Can you work these out from the drawing? Everything is in mm from the part's minimum corner. Coordinates: 2 decimals unless noted, no trailing zeros. Write each loop counter-clockwise with the first axis right and the second up, starting at its lowest first coordinate (ties: lowest second). Pieces come first, ordered by that corner, then holes. Notation, with made-up numbers: (54, 68) - (95, 68) arc R27 cw to (95, 96) - close; hole circle Ø3 at (57.5, -14.5). An arc over 180 degrees is marked (long way). One line per question, with ' | ' between items. Start each with the question number.
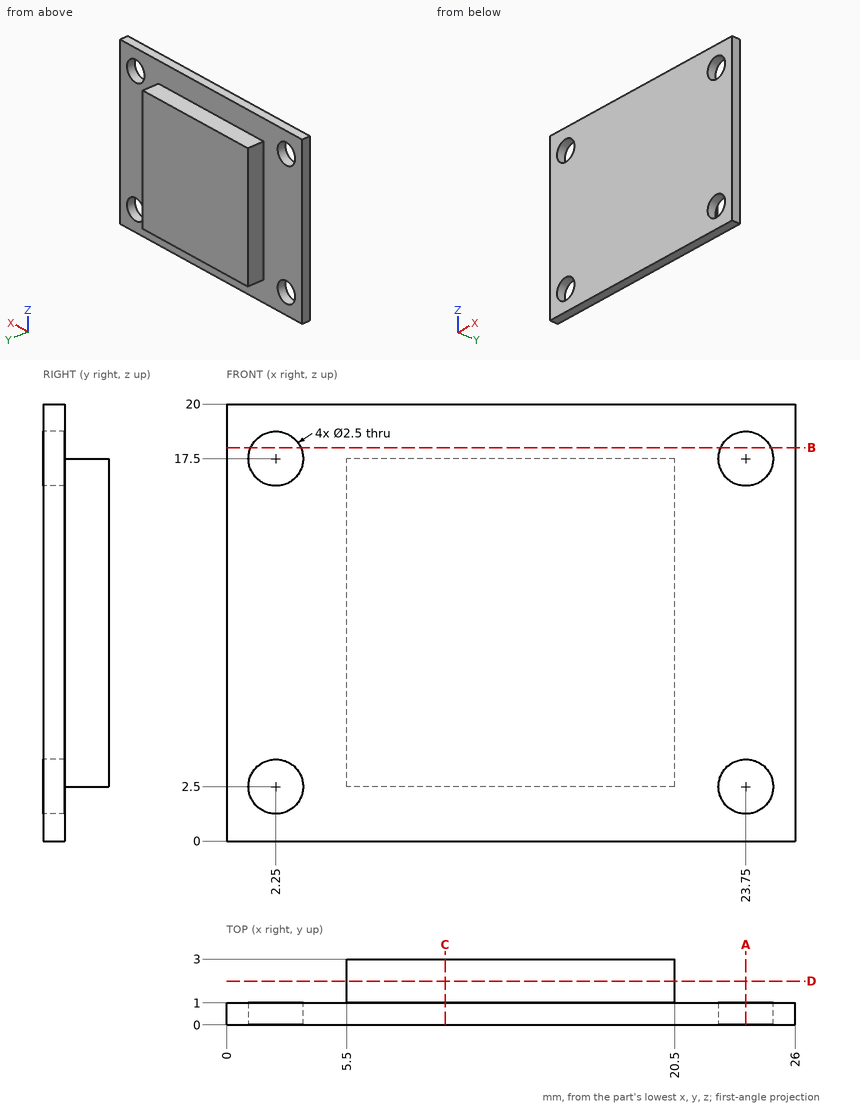
(1) I'm going to push flat-ended pins straight in: pin 1 (3 mm diameter, centred on x = 2.25, z = 17.5, fed in from +Y); pin 2 (1 mm diameter, centred on x = 10, y = 2, fed in from -Z); pin 3 (0.6 mm diameter, centred on y = 1.5, z = 10.5, fed in from -X). Where does each tip first touch, or does it pass through?
(2) If we section it at C-C on x = 10: List the corners of the cut face in (y, z) for me.
(3) If we section it at D-D on y = 2: List the corners of the cut face in (x, z) for me.
(4) If we section it at A-A on x = 23.75: List the corners of the cut face in (y, z) for me.
(5) If we section it at B-B on z = 18: List the corners of the cut face in (x, y) for me, plus the area to 3 significant figures.
(6) If I drill on probe 1 along Z at (x, y) = (2.25, 0.6); probe 2 along X at (y, z) = (0.5, 2.5); probe 3 along X at (y, z) = (1.75, 4.5), over which ranges is the centre line in solid material (lowest first)?
Values:
1) pin 1: y = 1 | pin 2: z = 2.5 | pin 3: x = 5.5
2) outline: (0, 0) - (1, 0) - (1, 2.5) - (3, 2.5) - (3, 17.5) - (1, 17.5) - (1, 20) - (0, 20) - close
3) outline: (5.5, 2.5) - (20.5, 2.5) - (20.5, 17.5) - (5.5, 17.5) - close
4) outline: (0, 0) - (1, 0) - (1, 1.25) - (0, 1.25) - close; (0, 3.75) - (1, 3.75) - (1, 16.25) - (0, 16.25) - close; (0, 18.75) - (1, 18.75) - (1, 20) - (0, 20) - close
5) outline: (0, 0) - (1.1, 0) - (1.1, 1) - (0, 1) - close; (3.4, 0) - (22.6, 0) - (22.6, 1) - (3.4, 1) - close; (24.9, 0) - (26, 0) - (26, 1) - (24.9, 1) - close | area: 21.4 mm2
6) probe 1: 0 to 1.25, 3.75 to 16.25, 18.75 to 20 | probe 2: 0 to 1, 3.5 to 22.5, 25 to 26 | probe 3: 5.5 to 20.5
